CAD build for the part. Positions are in the model's coordinates, mm. A direction names the side the tool comes from. Round coordinates to 2 decimals unless told otherwise and drop trailing zeros. Write each loop counter-clockwise with the first axis right and the second up, starting at its lowest first coordinate (ties: lowest second). Pieces come first, ordered by that corner, then holes. Notation, with made-up numbers: (39.5, 84.25) - (98.5, 84.25) arc R26 ccw to (98.5, 104.25) - close; hole circle Ø10 at (57, 49.25). An arc over 180 degrees is marked (long way). Use one line per item in the form item = value. Start each with the question number.
Item 1: Tool access for faces 1 (the flat face through (3.9, -2, 25)), 2 (the flat face through (0, 5, 60)), 3 (the flat face through (-3.9, -2, 25)), 4 (the flat face through (0, -3, 50)): list every direction of +Z, -Z, +X, -X, +Y, -Y with a clear straight run to the whole face (end or side of a thin tool).
Item 2: Drill centre lines: L1, parallel to Z at x = 0.75, y = -0.5; L2, parallel to X at y = 0.25, z = 40.5; L3, parallel to Y at x = -2.25, z = 56.5. Where is each one in solid material? Low to high.
Item 3: Band-saw the part on C-C, the plane x = 6. List the corners of the cut face in (y, z), and give its area (3 significant figures).
Item 4: Band-saw the part on A-A, the plane z = 23.5. List the corners of the cut face in (x, y).
Item 5: Pin check, flat tips, straight feed: pin 1 (5 mm diameter, centred on y = -1.5, z = 38.5, fed in from -X); pin 2 (2.5 mm diameter, centred on y = 0, z = 19, fed in from +X). Stop position of each tip, or through.
Item 6: Band-saw the part on D-D, the plane z = 55. List the corners of the cut face in (x, y), and give its area (3 significant figures).
Item 7: Band-saw the part on B-B, the plane y = 6.5. List the corners of the cut face in (x, z), and give its area (3 significant figures).
from build123d import *

# Parameters (mm, degrees)
BOX016_W                 = 16
BOX016_H                 = 6
BOX016_DEPTH             = 60
CHAMFER002001016_SIZE    = 3
BOX017_W                 = 7.8
BOX017_H                 = 10
BOX017_DEPTH             = 50
CHAMFER002001017_1_SIZE2 = 1
CHAMFER002001017_1_SIZE  = 2
CHAMFER002001017_2_SIZE2 = 1
CHAMFER002001017_2_SIZE  = 2
CHAMFER002001018_SIZE    = 0.4


with BuildPart() as chamfer002001016:
    # Box016 → Box016 (new body)
    with BuildSketch(Plane(origin=(-8, 2, 0), x_dir=(1, 0, 0), z_dir=(0, 0, 1))):
        with Locations((8, 3)):
            Rectangle(BOX016_W, BOX016_H)
    extrude(amount=BOX016_DEPTH)

    # Chamfer002001016
    chamfer002001016_edges = [chamfer002001016.edges().sort_by_distance(p)[0] for p in [
        (-8, 8, 30),
        (8, 8, 30),
    ]]
    chamfer(chamfer002001016_edges, length=CHAMFER002001016_SIZE)


with BuildPart() as chamfer002001018:
    # Box017 → Box017 (new body)
    with BuildSketch(Plane(origin=(-3.9, -8, 0), x_dir=(1, 0, 0), z_dir=(0, 0, 1))):
        with Locations((3.9, 5)):
            Rectangle(BOX017_W, BOX017_H)
    extrude(amount=BOX017_DEPTH)

    # Chamfer002001017 1
    chamfer002001017_1_edges = [chamfer002001018.edges().sort_by_distance(p)[0] for p in [
        (3.9, -8, 25),
    ]]
    chamfer002001017_1_side = chamfer002001018.faces().sort_by_distance((3.9, -3, 25))[0]
    chamfer(chamfer002001017_1_edges, length=CHAMFER002001017_1_SIZE, length2=CHAMFER002001017_1_SIZE2, reference=chamfer002001017_1_side)

    # Chamfer002001017 2
    chamfer002001017_2_edges = [chamfer002001018.edges().sort_by_distance(p)[0] for p in [
        (-3.9, -8, 25),
    ]]
    chamfer002001017_2_side = chamfer002001018.faces().sort_by_distance((-3.9, -3, 25))[0]
    chamfer(chamfer002001017_2_edges, length=CHAMFER002001017_2_SIZE, length2=CHAMFER002001017_2_SIZE2, reference=chamfer002001017_2_side)

    # Fusion003012003003: union Chamfer002001016
    add(chamfer002001016.part)

    # Chamfer002001018
    chamfer002001018_edges = [chamfer002001018.edges().sort_by_distance(p)[0] for p in [
        (-8, 2, 30),
        (8, 2, 30),
        (3.9, -6, 25),
        (-2.9, -8, 25),
        (2.9, -8, 25),
    ]]
    chamfer(chamfer002001018_edges, length=CHAMFER002001018_SIZE)


solid = chamfer002001018.part
Determined:
q1.face_1 = +Z, -Z, +X, -Y
q1.face_2 = +Z, +X, -X, +Y, -Y
q1.face_3 = +Z, -Z, -X, -Y
q1.face_4 = +Z, +X, -X, -Y
q2.L1 = 0 to 50
q2.L2 = -3.9 to 3.9
q2.L3 = 2 to 8
q3.outline = (2, 0) - (7, 0) - (7, 60) - (2, 60) - close
q3.area = 300 mm²
q4.outline = (-8, 2.4) - (-7.6, 2) - (-3.9, 2) - (-3.9, -6) - (-3.08, -7.64) - (-2.5, -8) - (2.5, -8) - (3.08, -7.64) - (3.72, -6.36) - (3.9, -5.6) - (3.9, 2) - (7.6, 2) - (8, 2.4) - (8, 5) - (5, 8) - (-5, 8) - (-8, 5) - close
q5.pin_1 = -3.9
q5.pin_2 = 3.9
q6.outline = (-8, 2.4) - (-7.6, 2) - (7.6, 2) - (8, 2.4) - (8, 5) - (5, 8) - (-5, 8) - (-8, 5) - close
q6.area = 86.8 mm²
q7.outline = (-6.5, 0) - (6.5, 0) - (6.5, 60) - (-6.5, 60) - close
q7.area = 780 mm²
